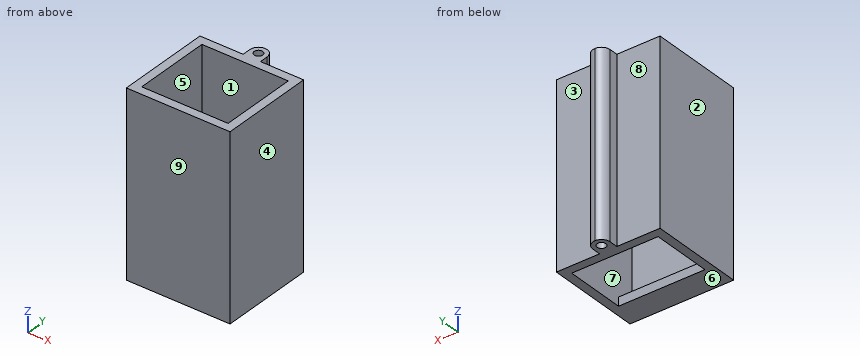
```python
from build123d import *

# Parameters (mm, degrees)
SKETCH3_W           = 60
SKETCH3_H           = 55
SKETCH3_W_2         = 50
SKETCH3_H_2         = 45
BOSS_EXTRUDE1_DEPTH = 105
SKETCH6_W           = 50
SKETCH6_H           = 5
BOSS_EXTRUDE3_DEPTH = 10
SKETCH7_W           = 10
SKETCH7_H           = 105
BOSS_EXTRUDE4_DEPTH = 10
FILLET1_R           = 5
SKETCH8_R           = 2.5
CUT_EXTRUDE1_DEPTH  = 116.461032388


with BuildPart() as part:
    # Sketch3 → Boss-Extrude1 (new body)
    with BuildSketch(Plane.XY):
        Rectangle(SKETCH3_W, SKETCH3_H)
        Rectangle(SKETCH3_W_2, SKETCH3_H_2, mode=Mode.SUBTRACT)
    extrude(amount=-BOSS_EXTRUDE1_DEPTH)

    # Sketch6 → Boss-Extrude3 (add)
    with BuildSketch(Plane(origin=(0, -22.5, 0), x_dir=(1, 0, 0), z_dir=(0, 1, 0))):
        with Locations((0, 102.5)):
            Rectangle(SKETCH6_W, SKETCH6_H)
    extrude(amount=BOSS_EXTRUDE3_DEPTH)

    # Sketch7 → Boss-Extrude4 (add)
    with BuildSketch(Plane(origin=(0, 27.5, 0), x_dir=(1, 0, 0), z_dir=(0, 1, 0))):
        with Locations((0, 52.5)):
            Rectangle(SKETCH7_W, SKETCH7_H)
    extrude(amount=BOSS_EXTRUDE4_DEPTH)

    # Fillet1
    fillet1_edges = [part.edges().sort_by_distance(p)[0] for p in [
        (5, 37.5, -52.5),
        (-5, 37.5, -52.5),
    ]]
    fillet(fillet1_edges, radius=FILLET1_R - 0.0001)  # a hair under: the kernel refuses the full size

    # Sketch8 → Cut-Extrude1 (cut, through all)
    with BuildSketch(Plane.XY):
        with Locations((0, 32.5)):
            Circle(SKETCH8_R)
    extrude(amount=-CUT_EXTRUDE1_DEPTH, mode=Mode.SUBTRACT)


solid = part.part
```
Work out the finished part from the listing and answer in its coordinate system (mm). Face numbers are marked on the shaded views. A direction names the side the tool comes from. Coordinates: 2 decimals unless noted, no trailing zeros. Loops run counter-clockwise (first coordinate to the right, second up) from the corner with the lowest first, then second, coordinate; pieces in that order, holes last.
1) Section C-C (z = -60) is taken. Give the number of separate pieces and of enclosed holes in the cut face, plus the area to 3 significant figures.
Results:
separate pieces: 1
enclosed holes: 2
area: 1,120 mm2
2) For a pull along Y with two mould halves and no side action, classify the marked faces 6, 7, 8 and 9 as +Y half, -Y half, draft (parallel to the pull), parting line (faces both ways), or undercut.
Results:
face 6: draft
face 7: undercut
face 8: +Y half
face 9: -Y half
3) For the marked faces 1, 2, 3, 4 and 5, determine the directions among +Z, -Z, +X, -X, +Y, -Y from which every point of the face is accessible in a straight line to the end or side of a thin tool.
Results:
face 1: +Z, -Z
face 2: +Z, -Z, -X, +Y, -Y
face 3: +Z, -Z, +X, +Y
face 4: +Z, -Z, +X, +Y, -Y
face 5: +Z
4) Flat-ended cylindrical pins translate along their axes: pin 1 (8 mm diameter, centred on x = -13.5, z = -61, fed in from +Y); pin 2 (2.5 mm diameter, centred on y = 30.5, z = -63, fed in from +X); pin 3 (6.5 mm diameter, centred on x = 0, y = 32.5, fed in from -Z); pin 4 (8 mm diameter, centred on x = -10.5, y = -16.5, fed in from +Z). Find the tip coordinate at first contact, or state that the pin passes through.
Results:
pin 1: stops at y = 27.5
pin 2: stops at x = 5
pin 3: stops at z = -105
pin 4: stops at z = -100
5) Consider probe 1 along Y at (x, z) = (0, -81); probe 2 along Y at (x, z) = (19, -28); probe 3 along X at (y, z) = (1, -77). Determine where each line is inside the solid, lowest interval first.
Results:
probe 1: y = -27.5 to -22.5, 22.5 to 30, 35 to 37.5
probe 2: y = -27.5 to -22.5, 22.5 to 27.5
probe 3: x = -30 to -25, 25 to 30
6) Section D-D (y = -20.5) is taken. Give the vertices of the cut face in (x, z), plus the area to 3 significant figures.
Results:
outline: (-30, -105) - (30, -105) - (30, 0) - (25, 0) - (25, -100) - (-25, -100) - (-25, 0) - (-30, 0) - close
area: 1,300 mm2
7) Section B-B (x = -14) is taken. Give the vertices of the cut face in (y, z).
Results:
outline: (-27.5, -105) - (-12.5, -105) - (-12.5, -100) - (-22.5, -100) - (-22.5, 0) - (-27.5, 0) - close; (22.5, -105) - (27.5, -105) - (27.5, 0) - (22.5, 0) - close
8) Section A-A (y = 19.5) is taken. Give the vertices of the cut face in (x, z).
Results:
outline: (-30, -105) - (-25, -105) - (-25, 0) - (-30, 0) - close; (25, -105) - (30, -105) - (30, 0) - (25, 0) - close
